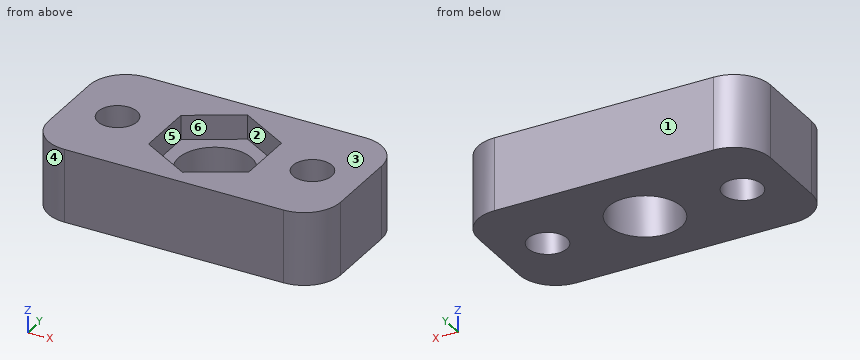
```python
from build123d import *

# Parameters (mm, degrees)
SKETCH_W          = 24
SKETCH_H          = 12
SKETCH_R          = 3
PAD_DEPTH         = 4
SKETCH001_W       = 24
SKETCH001_H       = 12
PAD001_DEPTH      = 2
SKETCH002_R       = 1.6
POCKET_DEPTH      = 4.001
POCKET_DEPTH_BACK = -2.001
FILLET_R          = 3


with BuildPart() as part:
    # Sketch → Pad (new body)
    with BuildSketch(Plane.XY):
        Rectangle(SKETCH_W, SKETCH_H)
        Circle(SKETCH_R, mode=Mode.SUBTRACT)
    extrude(amount=-PAD_DEPTH)

    # Sketch001 → Pad001 (join)
    with BuildSketch(Plane.XY):
        Rectangle(SKETCH001_W, SKETCH001_H)
        Polygon((4.125, -2.38157), (4.125, 2.38157), (0, 4.76314), (-4.125, 2.38157), (-4.125, -2.38157), (0, -4.76314), align=None, mode=Mode.SUBTRACT)
    extrude(amount=PAD001_DEPTH)

    # Sketch002 → Pocket (cut, two sides)
    with BuildSketch(Plane.XY) as pocket_sk:
        with Locations((-8, 0)):
            Circle(SKETCH002_R)
        with Locations((8, 0)):
            Circle(SKETCH002_R)
    extrude(amount=-POCKET_DEPTH, mode=Mode.SUBTRACT)
    extrude(pocket_sk.sketch, amount=-POCKET_DEPTH_BACK, mode=Mode.SUBTRACT)

    # Fillet
    fillet_edges = [part.edges().sort_by_distance(p)[0] for p in [
        (-12, -6, -2),
        (-12, 6, -2),
        (12, 6, -2),
        (12, -6, -2),
    ]]
    fillet(fillet_edges, radius=FILLET_R)


solid = part.part
```
CAD build for the part. Positions are in the model's coordinates, mm. Face numbers are marked on the shaded views. A direction names the side the tool comes from. Round coordinates to 2 decimals unless told otherwise and drop trailing zeros. Write each loop counter-clockwise with the first axis right and the second up, starting at its lowest first coordinate (ties: lowest second). Pieces come first, ordered by that corner, then holes. Notation, with made-up numbers: M 13.25,31 L 54.25,31 A20 cw 54.25,45 Z; hole C -32.5,88 d3. An arc over 180 degrees is marked long. One line per question, with ' | ' between items.
1. Cut at A-A on z = 1.65. Write the cut outline in (x, y) (3 decimals), and give its area (3 significant figures).
Working result:
outline: M -12,-3 A3 ccw -9,-6 L 9,-6 A3 ccw 12,-3 L 12,3 A3 ccw 9,6 L -9,6 A3 ccw -12,3 Z; hole C -8,0 d3.2; hole M -4.125,-2.382 L 0,-4.763 L 4.125,-2.382 L 4.125,2.382 L 0,4.763 L -4.125,2.382 Z; hole C 8,0 d3.2 | area: 205 mm2
2. Cut at B-B on x = -8. Write the cut outline in (y, z), and give its area (3 significant figures).
Working result:
outline: M -6,-4 L -1.6,-4 L -1.6,2 L -6,2 Z; M 1.6,-4 L 6,-4 L 6,2 L 1.6,2 Z | area: 52.8 mm2
3. Mould opens along X. For the marked faces 3, 4, 5 and 6 say: pulls with the +X half, pulls with the -X half, needs draft (parallel to the pull), parting line crosses it, or undercut.
Working result:
face 3: needs draft | face 4: pulls with the -X half | face 5: undercut | face 6: undercut
4. Cut at D-D on z = -0.95. Write the cut outline in (x, y), and give its area (3 significant figures).
Working result:
outline: M -12,-3 A3 ccw -9,-6 L 9,-6 A3 ccw 12,-3 L 12,3 A3 ccw 9,6 L -9,6 A3 ccw -12,3 Z; hole C -8,0 d3.2; hole C 0,0 d6; hole C 8,0 d3.2 | area: 236 mm2
5. Pin check, flat tips, straight feed: pin 1 Ø1.9 at (x, y) = (8, 0) entering from -Z; pin 2 Ø2.5 at (x, y) = (-1.5, -1) entering from +Z; pin 3 Ø4 at (x, y) = (-8, 0) entering from -Z. Stop position of each tip, or through.
Working result:
pin 1: through | pin 2: z = 0 | pin 3: z = -4
6. Which spindle directions (+Z, -Z, +X, -X, +Y, -Y) get a long thin tool onto all of the face, cutting with end or side? Do the marked faces 1 and 2. Say none if no direction does.
Working result:
face 1: +Z, -Z, +X, -X, +Y | face 2: +Z
7. Cut at C-C on y = 0. Write the cut outline in (x, z) (3 decimals).
Working result:
outline: M -12,-4 L -9.6,-4 L -9.6,2 L -12,2 Z; M -6.4,-4 L -3,-4 L -3,0 L -4.125,0 L -4.125,2 L -6.4,2 Z; M 3,-4 L 6.4,-4 L 6.4,2 L 4.125,2 L 4.125,0 L 3,0 Z; M 9.6,-4 L 12,-4 L 12,2 L 9.6,2 Z
8. Probe L1, parallel to X at y = 0, z = 0.7 (3 decimals); L2, parallel to Y at x = 8, z = 0.9; L3, parallel to Y at x = 1, z = -2.3. List the from-to ranges inside material, lowest first. Write a range as from..to.
Working result:
L1: -12..-9.6, -6.4..-4.125, 4.125..6.4, 9.6..12 | L2: -6..-1.6, 1.6..6 | L3: -6..-2.83, 2.83..6
